Can you work these out from the drawing? Everything is in mm from the part's minimum corner. A direction names the side the tool comes from. Round coordinates to 2 decimals unless told otherwise and drop trailing zeros. Loops run counter-clockwise (first coordinate to the right, second up) from the corner with the lowest first, then second, coordinate; pieces in that order, holes last. Notation, with made-up numbers: M 48,2 L 74,2 A34 ccw 74,36 Z; hole C 4,-19 d6. An arc over 180 degrees is marked long. Use a Markdown table: item, result.
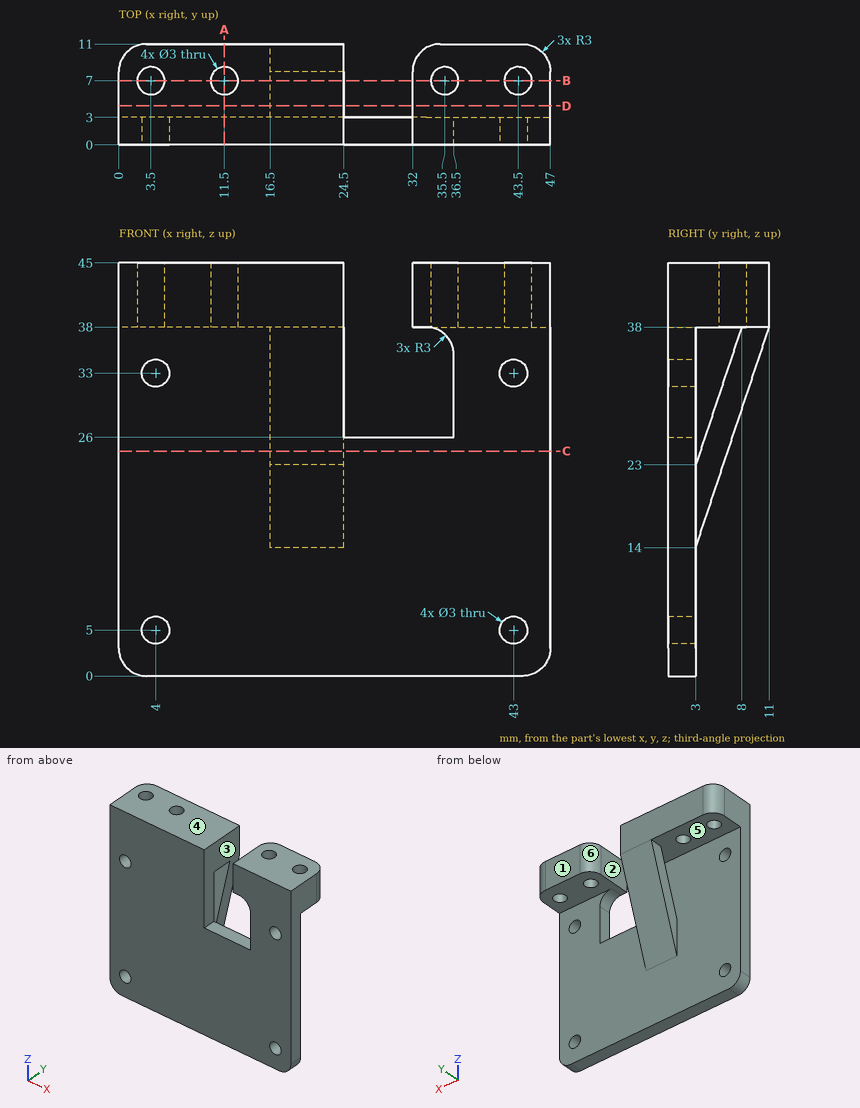
Q1. For the marked faces 1, 2 and 3, which set-ups out of +Z, -Z, +X, -X, +Y, -Y let a thin tool reach every point of the face, with its end or its side?
Return value:
| item | result |
|---|---|
| face 1 | +Z, -Z, +X, -X, +Y |
| face 2 | +Z, +Y, -Y |
| face 3 | +Z, +Y |
Q2. Imagine slicing it at A-A, the plane x = 11.5. Please give me the cut outline in (y, z), then the cut area to 3 significant figures.
Return value:
| item | result |
|---|---|
| outline | M 0,0 L 3,0 L 3,38 L 5.5,38 L 5.5,45 L 0,45 Z; M 8.5,38 L 11,38 L 11,45 L 8.5,45 Z |
| area | 170 mm^2 |
Q3. Imagine slicing it at B-B, the plane y = 7. Please give me the cut outline in (x, z), then the cut area to 4 significant figures.
Return value:
| item | result |
|---|---|
| outline | M 0,38 L 2,38 L 2,45 L 0,45 Z; M 5,38 L 10,38 L 10,45 L 5,45 Z; M 13,38 L 24.5,38 L 24.5,45 L 13,45 Z; M 16.5,26 L 24.5,26 L 24.5,35 L 16.5,35 Z; M 32,38 L 34,38 L 34,45 L 32,45 Z; M 37,38 L 42,38 L 42,45 L 37,45 Z; M 45,38 L 47,38 L 47,45 L 45,45 Z |
| area | 264.5 mm^2 |
Q4. Imagine slicing it at D-D, the plane y = 4.25. Please give me the cut outline in (x, z), then the cut area to 4 significant figures.
Return value:
| item | result |
|---|---|
| outline | M 0,38 L 24.5,38 L 24.5,45 L 0,45 Z; M 16.5,17.75 L 24.5,17.75 L 24.5,26.75 L 16.5,26.75 Z; M 32,38 L 47,38 L 47,45 L 32,45 Z |
| area | 348.5 mm^2 |
Q5. We'd pull the mould along Y, two halves only. Please class the marked faces 4, 5 and 6: pulls with the +Y half, pulls with the -Y half, needs draft (parallel to the pull), parting line crosses it, or undercut.
Return value:
| item | result |
|---|---|
| face 4 | needs draft |
| face 5 | undercut |
| face 6 | pulls with the +Y half |
Q6. I need wall thicknesses on line 1 (X direction, y = 2, z = 5); line 2 (X direction, y = 0.85, z = 33); line 3 (X direction, y = 3.5, z = 42.5). Which ranges of each line are inside material? Lowest first, please. Write a range as from..to.
Return value:
| item | result |
|---|---|
| line 1 | x = 0..2.5, 5.5..41.5, 44.5..47 |
| line 2 | x = 0..2.5, 5.5..24.5, 36.5..41.5, 44.5..47 |
| line 3 | x = 0..24.5, 32..47 |
Q7. Imagine slicing it at C-C, the plane z = 24.5. Please give me the cut outline in (x, y).
Return value:
| item | result |
|---|---|
| outline | M 0,0 L 47,0 L 47,3 L 0,3 Z; M 16.5,3.5 L 24.5,3.5 L 24.5,6.5 L 16.5,6.5 Z |
Q8. Will these pins go through, and if not, where does the flat tip stop? P1, Ø4, axis at x = 43, z = 5, coming from the +Y side; P2, Ø1.5, axis at y = 9.5, z = 39, coming from the +X side; P3, Ø4, axis at x = 21.5, z = 30.5, coming from the +Y side.
Return value:
| item | result |
|---|---|
| P1 | stops at y = 3 |
| P2 | stops at x = 46.9 |
| P3 | stops at y = 9.17 |
